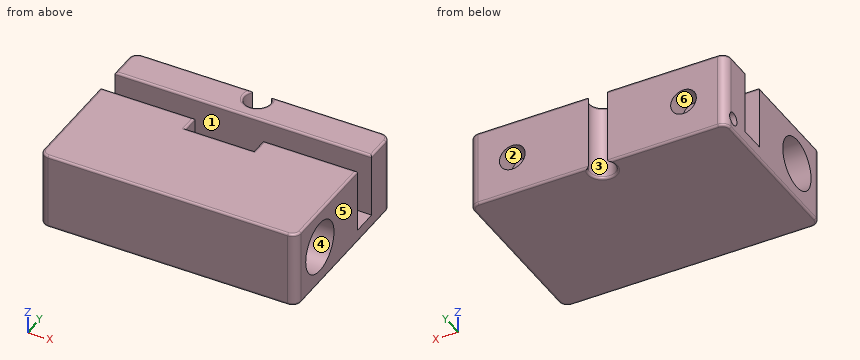
```python
from build123d import *

# Parameters (mm, degrees)
SKETCH1_W           = 60
SKETCH1_H           = 40
BOSS_EXTRUDE1_DEPTH = 9
SKETCH2_R           = 6
CUT_EXTRUDE1_DEPTH  = 64.882705015
SKETCH3_R           = 3
CUT_EXTRUDE2_DEPTH  = 41.298883359
CUT_EXTRUDE3_DEPTH  = 15
SKETCH5_R           = 1
CUT_EXTRUDE4_DEPTH  = 29
SKETCH6_R           = 1.5
CUT_EXTRUDE5_DEPTH  = 5
CUT_EXTRUDE6_REACH  = 52.804
SKETCH7_R           = 2
SKETCH8_R           = 3
CUT_EXTRUDE7_DEPTH  = 5
FILLET1_R           = 2
FILLET2_R           = 0.5


with BuildPart() as part:
    # Sketch1 → Boss-Extrude1 (new, symmetric)
    with BuildSketch(Plane.XY):
        Rectangle(SKETCH1_W, SKETCH1_H)
    extrude(amount=BOSS_EXTRUDE1_DEPTH, both=True)

    # Sketch2 → Cut-Extrude1 (cut, through all)
    with BuildSketch(Plane.ZY.offset(30)):
        with Locations(Location((0, -10, 0), (0, 0, 270))):
            Circle(SKETCH2_R)
    extrude(amount=-CUT_EXTRUDE1_DEPTH, mode=Mode.SUBTRACT)

    # Sketch3 → Cut-Extrude2 (cut, through all)
    with BuildSketch(Plane.XY.offset(9)):
        with Locations((0, 18)):
            Circle(SKETCH3_R)
    extrude(amount=-CUT_EXTRUDE2_DEPTH, mode=Mode.SUBTRACT)

    # Sketch4 → Cut-Extrude3 (cut)
    with BuildSketch(Plane.XY.offset(9)):
        Polygon((-30, 12), (30, 12), (30, 6), (8, 6), (8, 2), (-8, 2), (-8, 6), (-30, 6), align=None)
    extrude(amount=-CUT_EXTRUDE3_DEPTH, mode=Mode.SUBTRACT)

    # Sketch5 → Cut-Extrude4 (cut)
    with BuildSketch(Plane.ZY.offset(30)):
        with Locations(Location((-6, 17, 0), (0, 0, 270))):
            Circle(SKETCH5_R)
    extrude(amount=-CUT_EXTRUDE4_DEPTH, mode=Mode.SUBTRACT)

    # Sketch6 → Cut-Extrude5 (cut)
    with BuildSketch(Plane.ZY.offset(30)):
        with Locations(Location((-6, 17, 0), (0, 0, 270))):
            Circle(SKETCH6_R)
    extrude(amount=-CUT_EXTRUDE5_DEPTH, mode=Mode.SUBTRACT)

    # Sketch7 → Cut-Extrude6 (cut, up to next)
    with BuildSketch(Plane(origin=(0, 20, 0), x_dir=(1, 0, 0), z_dir=(0, 1, 0)), mode=Mode.PRIVATE) as cut_extrude6_sk1:
        with Locations(Location((-20, 0, 0), (0, 0, 270))):
            Circle(SKETCH7_R)
    cut_extrude6_tool1 = extrude(cut_extrude6_sk1.sketch, amount=-CUT_EXTRUDE6_REACH, mode=Mode.PRIVATE) & part.part
    # Sketch7 → Cut-Extrude6 (cut, up to next)
    with BuildSketch(Plane(origin=(0, 20, 0), x_dir=(1, 0, 0), z_dir=(0, 1, 0)), mode=Mode.PRIVATE) as cut_extrude6_sk2:
        with Locations(Location((20, 0, 0), (0, 0, 270))):
            Circle(SKETCH7_R)
    cut_extrude6_tool2 = extrude(cut_extrude6_sk2.sketch, amount=-CUT_EXTRUDE6_REACH, mode=Mode.PRIVATE) & part.part
    add(cut_extrude6_tool1.solids().sort_by_distance((-20, 20, 0))[0], mode=Mode.SUBTRACT)
    add(cut_extrude6_tool2.solids().sort_by_distance((20, 20, 0))[0], mode=Mode.SUBTRACT)

    # Sketch8 → Cut-Extrude7 (cut)
    with BuildSketch(Plane(origin=(0, 20, 0), x_dir=(1, 0, 0), z_dir=(0, 1, 0))):
        with Locations(Location((-20, 0, 0), (0, 0, 270))):
            Circle(SKETCH8_R)
        with Locations(Location((20, 0, 0), (0, 0, 90))):
            Circle(SKETCH8_R)
    extrude(amount=-CUT_EXTRUDE7_DEPTH, mode=Mode.SUBTRACT)

    # Fillet1
    # the kernel refuses this fillet: 2 mm, written as the material it takes off along each edge
    with BuildSketch(Plane(origin=(30, -20, 14), x_dir=(-1, 0, 0), z_dir=(0, 0, -1))) as fillet1_piece_1:
        with BuildLine():
            CenterArc((FILLET1_R, FILLET1_R), FILLET1_R, 180, 90)
            Line((0, FILLET1_R), (0, 0))
            Line((0, 0), (FILLET1_R, 0))
        make_face()
    extrude(amount=28, mode=Mode.SUBTRACT)
    with BuildSketch(Plane(origin=(-30, -20, -14), x_dir=(0, 1, 0), z_dir=(0, 0, 1)), Plane(origin=(-30, 20, -14), x_dir=(1, 0, 0), z_dir=(0, 0, 1)), Plane(origin=(30, 20, 14), x_dir=(-1, 0, 0), z_dir=(0, 0, -1))) as fillet1_piece_2:
        with BuildLine():
            CenterArc((FILLET1_R, -FILLET1_R), FILLET1_R, 90, 90)
            Line((0, -FILLET1_R), (0, 0))
            Line((0, 0), (FILLET1_R, 0))
        make_face()
    extrude(amount=28, mode=Mode.SUBTRACT)

    # Fillet2
    fillet2_edges = [part.edges().sort_by_distance(p)[0] for p in [
        (29.414213562, -19.414213562, 9),
        (15.118033989, 20, 9),
        (-30, 15, 9),
        (-29.414213562, 19.414213562, 9),
        (29.414213562, 19.414213562, 9),
        (-15.118033989, 20, -9),
        (0, 15, -9),
        (-15.118033989, 20, 9),
        (0, 15, 9),
        (-30, -6, 9),
        (30, 15, 9),
        (-19, 6, 9),
        (-8, 4, 9),
        (0, 2, 9),
        (8, 4, 9),
        (19, 6, 9),
        (0, 12, 9),
        (30, -6, 9),
        (30, 0, -9),
        (15.118033989, 20, -9),
        (0, -20, -9),
        (-30, 0, -9),
        (-29.414213562, 19.414213562, -9),
        (-29.414213562, -19.414213562, -9),
        (29.414213562, 19.414213562, -9),
        (29.414213562, -19.414213562, -9),
        (0, -20, 9),
        (-29.414213562, -19.414213562, 9),
    ]]
    fillet(fillet2_edges, radius=FILLET2_R)


solid = part.part
```
CAD build for the part. Positions are in the model's coordinates, mm. Face numbers are marked on the shaded views. A direction names the side the tool comes from. Give positions to 0.01 mm unless a question says otherwise; leave off trailing zeros. Order: outer loops, then holes, each group sorted by start corner. A loop starts at its lowest first (then second) coordinate and runs counter-clockwise, first axis right, second up.
(1) Saw through at D-D, the plane y = 7. Give the cut face in (x, z), then the cut area to 3 significant figures.
(2) Drill centre lines: L1, parallel to X at y = 12.9, z = 0; L2, parallel to Z at x = -13.5, y = 17; L3, parallel to Y at x = 1.5, z = -0.5. Where is each one in solid material? Low to high.
(3) Saw through at C-C, the plane x = 5. Give the cut face in (y, z).
(4) Tool access for the marked faces 1, 2 and 3: list every direction of +Z, -Z, +X, -X, +Y, -Y with a clear straight run to the whole face (end or side of a thin tool).
(5) Mould opens along X. For the marked faces 4, 5 and 6 say: released by +X, released by -X, zero draft, split by the parting line, or undercut.
(6) Saw through at A-A, the plane x = 20. Give the cut face in (y, z).
(7) Saw through at B-B, the plane x = -20. Give the cut face in (y, z), then the cut area to 3 significant figures.
(8) Flat gauge pins, fed straight in: pin 1 (3 mm diameter, centred on x = 14, y = 9.5, fed in from +Z); pin 2 (1.8 mm diameter, centred on x = -19.5, z = 0.5, fed in from +Y); pin 3 (2.5 mm diameter, centred on y = 17, z = -6, fed in from -X). Where does each tip first touch, or does it go through?
Results found:
1. outline: (-30, -8.5) arc R0.5 ccw to (-29.5, -9) - (29.5, -9) arc R0.5 ccw to (30, -8.5) - (30, -6) - (-30, -6) - close
1. area: 180 mm2
2. L1: x = -30 to -22, -18 to 18, 22 to 30
2. L2: z = -9 to -7, -5 to 9
2. L3: y = -20 to -15.98, -4.02 to 2, 12 to 15.4
3. outline: (-20, -8.5) arc R0.5 ccw to (-19.5, -9) - (19.5, -9) arc R0.5 ccw to (20, -8.5) - (20, 8.5) arc R0.5 ccw to (19.5, 9) - (12.5, 9) arc R0.5 ccw to (12, 8.5) - (12, -6) - (2, -6) - (2, 8.5) arc R0.5 ccw to (1.5, 9) - (-19.5, 9) arc R0.5 ccw to (-20, 8.5) - close; hole circle Ø12 at (-10, 0)
4. face 1: +Z, +X, -X
4. face 2: +Y
4. face 3: +Z, -Z
5. face 4: zero draft
5. face 5: released by +X
5. face 6: undercut
6. outline: (-20, -8.5) arc R0.5 ccw to (-19.5, -9) - (19.5, -9) arc R0.5 ccw to (20, -8.5) - (20, -3) - (15, -3) - (15, -2) - (12, -2) - (12, -6) - (6, -6) - (6, 8.5) arc R0.5 ccw to (5.5, 9) - (-19.5, 9) arc R0.5 ccw to (-20, 8.5) - close; (12, 2) - (15, 2) - (15, 3) - (20, 3) - (20, 8.5) arc R0.5 ccw to (19.5, 9) - (12.5, 9) arc R0.5 ccw to (12, 8.5) - close; hole circle Ø12 at (-10, 0)
7. outline: (-20, -8.5) arc R0.5 ccw to (-19.5, -9) - (19.5, -9) arc R0.5 ccw to (20, -8.5) - (20, -3) - (15, -3) - (15, -2) - (12, -2) - (12, -6) - (6, -6) - (6, 8.5) arc R0.5 ccw to (5.5, 9) - (-19.5, 9) arc R0.5 ccw to (-20, 8.5) - close; (12, 2) - (15, 2) - (15, 3) - (20, 3) - (20, 8.5) arc R0.5 ccw to (19.5, 9) - (12.5, 9) arc R0.5 ccw to (12, 8.5) - close; hole circle Ø12 at (-10, 0); hole circle Ø2 at (17, -6)
7. area: 471 mm2
8. pin 1: stops at z = -6
8. pin 2: stops at y = 6
8. pin 3: stops at x = -25
